```python
from build123d import *

# Parameters (mm, degrees)
SKETCH1_R           = 42.5
BOSS_EXTRUDE1_DEPTH = 100
BOSS_EXTRUDE2_DEPTH = 200
SKETCH5_W           = 160
SKETCH5_H           = 220
BOSS_EXTRUDE4_DEPTH = 12.5
SKETCH6_R           = 40
CUT_EXTRUDE1_DEPTH  = 250


with BuildPart() as part:
    # Sketch1 → Boss-Extrude1 (new body)
    with BuildSketch(Plane.XY):
        Circle(SKETCH1_R)
    extrude(amount=-BOSS_EXTRUDE1_DEPTH)

    # Sketch2 → Boss-Extrude2 (add)
    with BuildSketch(Plane(origin=(0, 0, -100), x_dir=(-1, 0, 0), z_dir=(0, 0, -1))):
        with BuildLine():
            Line((-42.5, 350), (42.5, 350))
            Line((42.5, 350), (42.5, 0))
            ThreePointArc((42.5, 0), (0, -42.5), (-42.5, 0))
            Line((-42.5, 0), (-42.5, 350))
        make_face()
    extrude(amount=BOSS_EXTRUDE2_DEPTH)

    # Sketch5 → Boss-Extrude4 (add, symmetric)
    with BuildSketch(Plane(origin=(0, 350, 104.422680699), x_dir=(1, 0, 0), z_dir=(0, 1, 0))):
        with Locations((0, 300)):
            Rectangle(SKETCH5_W, SKETCH5_H)
    extrude(amount=BOSS_EXTRUDE4_DEPTH, both=True)

    # Sketch6 → Cut-Extrude1 (cut)
    with BuildSketch(Plane(origin=(0, 362.5, 104.422680699), x_dir=(1, 0, 0), z_dir=(0, 1, 0))):
        with Locations((0, 300)):
            Circle(SKETCH6_R)
    extrude(amount=-CUT_EXTRUDE1_DEPTH, mode=Mode.SUBTRACT)


solid = part.part
```
Can you work these out from the model? Positions are in its coordinate system, mm. A direction names the side the tool comes from. Give positions to 0.01 mm unless a question says otherwise; leave off trailing zeros. Order: outer loops, then holes, each group sorted by start corner. A loop starts at its lowest first (then second) coordinate and runs counter-clockwise, first axis right, second up. Notation, with made-up numbers: M 73,43 L 118,43 A11 cw 118,58 Z; hole C 84.25,-17 d9. An arc over 180 degrees is marked long. One line per item, written item: value.
1) We'd pull the mould along Y, two halves only. Please class faces 4 (the face through (-5.207, 239.25, -235.237)), 5 (the face through (-1, 171, -100)), 6 (the face through (34, 362.5, -173)): released by +Y, released by -Y, zero draft, split by the parting line, or undercut.
Answer sheet:
face 4: zero draft
face 5: undercut
face 6: released by +Y
2) I want a section at B-B, the plane y = 21. List the corners of the cut face in (x, z) for me, plus the area to 3 significant figures.
Answer sheet:
outline: M -42.5,-300 L 42.5,-300 L 42.5,-100 L 36.95,-100 L 36.95,0 L -36.95,0 L -36.95,-100 L -42.5,-100 Z
area: 24,400 mm^2
3) For P1, Ø7.5, axis at x = 14.5, y = 352, coming from the +Z side; P2, Ø4, axis at x = -27, y = 123.5, coming from the +Z side; P3, Ø3, axis at y = 273.5, z = -222, coming from the -X side, each with a flat end and sliding along its axis, tell me the tip position at first contact or that it passes through.
Answer sheet:
P1: stops at z = -85.58
P2: stops at z = -100
P3: stops at x = -42.5
4) I want a section at A-A, the plane x = 0. List the corners of the cut face in (y, z) for me, plus the area to 3 significant figures.
Answer sheet:
outline: M -42.5,-300 L 337.5,-300 L 337.5,-305.58 L 362.5,-305.58 L 362.5,-235.58 L 112.5,-235.58 L 112.5,-155.58 L 362.5,-155.58 L 362.5,-85.58 L 337.5,-85.58 L 337.5,-100 L 42.5,-100 L 42.5,0 L -42.5,0 Z
area: 70,000 mm^2
5) I want a section at C-C, the plane y = 139.5. List the corners of the cut face in (x, z) for me.
Answer sheet:
outline: M -42.5,-300 L 42.5,-300 L 42.5,-100 L -42.5,-100 Z; hole C 0,-195.58 d80
6) I want a section at D-D, the plane x = -34.5. List the corners of the cut face in (y, z) for me.
Answer sheet:
outline: M -24.82,-300 L 337.5,-300 L 337.5,-305.58 L 362.5,-305.58 L 362.5,-215.82 L 112.5,-215.82 L 112.5,-175.34 L 362.5,-175.34 L 362.5,-85.58 L 337.5,-85.58 L 337.5,-100 L 24.82,-100 L 24.82,0 L -24.82,0 Z
7) Please list where these lines run through material, in increasing order: line 1 along Z through (x, y) = (0, 262); line 2 along X through (y, z) = (83, -233); line 3 along Y through (x, z) = (56, -268.5).
Answer sheet:
line 1: z = -300 to -235.58, -155.58 to -100
line 2: x = -42.5 to 42.5
line 3: y = 337.5 to 362.5
8) On a 3-axis mill with a long thin cutter (end or side, diameter ignored), from which of +Z, -Z, +X, -X, +Y, -Y can I reach the whole of each face in a straight line? I mean faces 1 (the face through (-42.5, 171, -199)), 2 (the face through (-1, 150, -300)), 3 (the face through (-1, 350, -85.577)). Say none if no direction works.
Answer sheet:
face 1: +Z, -Z, -X, -Y
face 2: -Z, +X, -X, -Y
face 3: +Z, +X, -X, +Y
